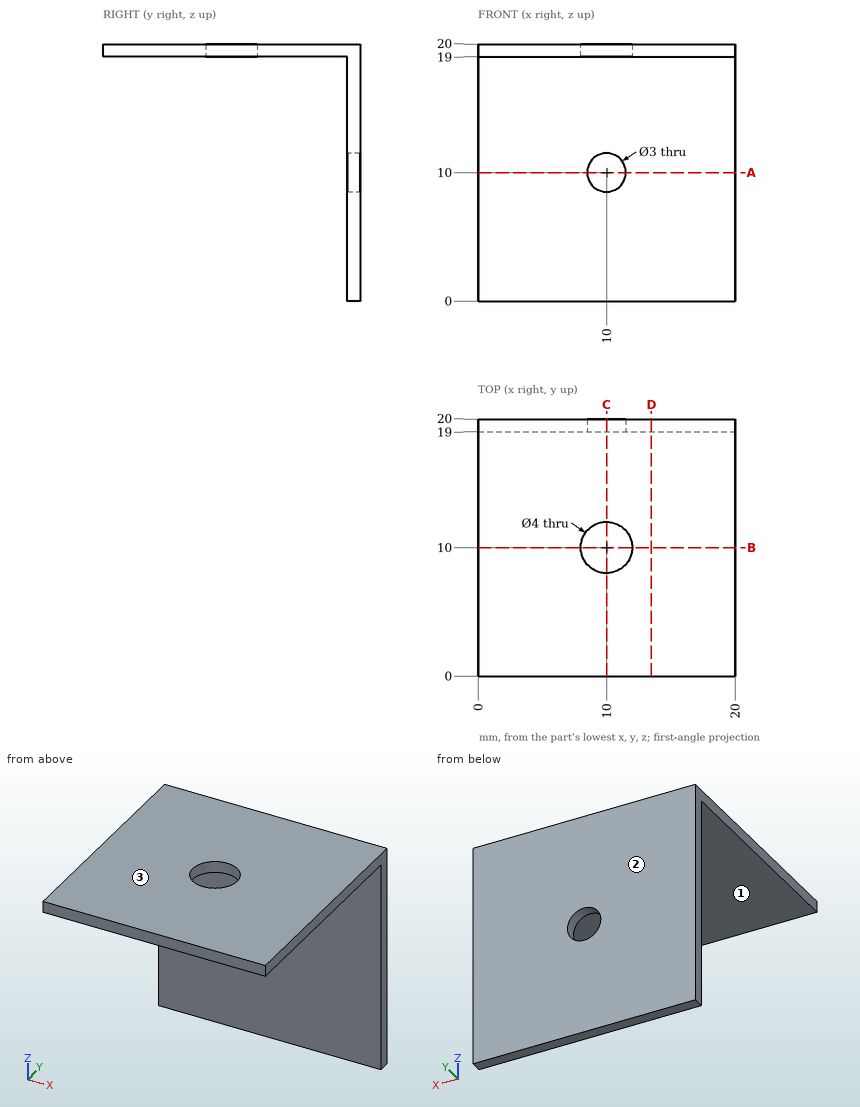
Geometry: see drawing. Coordinates: mm, zero at the bounding-box minimum. Give positions to 0.01 mm unless a question says otherwise; leave off trailing zeros. Write each loop counter-clockwise with the first axis right and the second up, starting at its lowest first coordinate (ties: lowest second). Pieces come first, ordered by that corner, then holes. Notation, with made-up numbers: M 52.5,2.25 L 71.5,2.25 A12 ccw 71.5,24.25 Z; hole C 11.25,-12.75 d10. An arc over 180 degrees is marked long. Answer as a JSON object with one key per item and string values.
Q1. Mould query, pull axis Z, two halves, no side actions, for the marked faces 1, 2 and 3. Classes: +Z half, -Z half, draft (parallel to the pull), parting line (faces both ways), or undercut.
Geometry check:
{"face 1": "-Z half", "face 2": "draft", "face 3": "+Z half"}
Q2. Cut plane B-B, the plane y = 10. Return the cut outline in (x, z).
Geometry check:
{"outline": "M 0,19 L 8,19 L 8,20 L 0,20 Z; M 12,19 L 20,19 L 20,20 L 12,20 Z"}
Q3. Ray query, line 1 along Y through (x, z) = (10, 19.5); line 2 along X through (y, z) = (19.55, 10); line 3 along Z through (x, y) = (6, 16.75). Return the intervals inside material, ascending.
Geometry check:
{"line 1": "y = 0 to 8, 12 to 20", "line 2": "x = 0 to 8.5, 11.5 to 20", "line 3": "z = 19 to 20"}
Q4. Contact query for flat-ended pins moving along their axis: P1, Ø10, axis at x = 17, z = 8.5, coming from the -Y side; P2, Ø5.5, axis at x = 11, y = 5, coming from the -Z side. Output: stop coordinate, or through.
Geometry check:
{"P1": "stops at y = 19", "P2": "stops at z = 19"}
Q5. Cut plane C-C, the plane x = 10. Return the cut outline in (y, z).
Geometry check:
{"outline": "M 0,19 L 8,19 L 8,20 L 0,20 Z; M 12,19 L 19,19 L 19,11.5 L 20,11.5 L 20,20 L 12,20 Z; M 19,0 L 20,0 L 20,8.5 L 19,8.5 Z"}
Q6. Cut plane A-A, the plane z = 10. Return the cut outline in (x, y).
Geometry check:
{"outline": "M 0,19 L 8.5,19 L 8.5,20 L 0,20 Z; M 11.5,19 L 20,19 L 20,20 L 11.5,20 Z"}
Q7. Cut plane D-D, the plane x = 13.5. Return the cut outline in (y, z).
Geometry check:
{"outline": "M 0,19 L 19,19 L 19,0 L 20,0 L 20,20 L 0,20 Z"}
